```python
from build123d import *

# Parameters (mm, degrees)
F0_R     = 100.5
F1_DEPTH = 107.5
F2_R     = 82
F3_DEPTH = 40
F5_DEPTH = 42.6


with BuildPart() as f1:
    # F0 (on Top) → F1 (new body)
    with BuildSketch(Plane.XY):
        Circle(F0_R)
    extrude(amount=F1_DEPTH)

    # F2 (on face) → F3 (join)
    with BuildSketch(Plane.XY.offset(107.5)):
        Circle(F2_R)
    extrude(amount=F3_DEPTH)

    # F4 (on face) → F5 (join)
    with BuildSketch(Plane(origin=(0, 0, 0), x_dir=(1, 0, 0), z_dir=(0, 0, -1))):
        with BuildLine():
            ThreePointArc((-2.4, 10.847677), (-6.955864, -8.663028), (11.11, 0))
            ThreePointArc((11.11, 0), (8.663028, 6.955864), (2.4, 10.847677))
            Line((2.4, 10.847677), (2.4, 8.46))
            Line((2.4, 8.46), (0, 8.46))
            Line((0, 8.46), (-2.4, 8.46))
            Line((-2.4, 8.46), (-2.4, 10.847677))
        make_face()
        with BuildLine():
            ThreePointArc((5.555, 0), (-3.927978, -3.927978), (0, 5.555))
            ThreePointArc((0, 5.555), (3.927978, 3.927978), (5.555, 0))
        make_face(mode=Mode.SUBTRACT)
    extrude(amount=F5_DEPTH)


solid = f1.part
```
Here's how the part is built. I have some questions about the finished solid (model axes, mm). A direction names the side the tool comes from. Coordinates: 2 decimals unless noted, no trailing zeros. Order: outer loops, then holes, each group sorted by start corner. A loop starts at its lowest first (then second) coordinate and runs counter-clockwise, first axis right, second up.
1) Which directions (+Z, -Z, +X, -X, +Y, -Y) give clear straight access to the entire face, cutting with the end or side of a thin tool? Please do faces 1 (the face through (0, 0, 0)), 2 (the face through (-3, -5, -42.6)), 3 (the face through (-82.4, 0.5, 107.5)).
2) Will these pins go through, and if not, where does the flat tip stop? pin 1 (2 mm diameter, centred on x = -58, z = 60.5, fed in from -Y); pin 2 (5.5 mm diameter, centred on x = 0.5, z = -19, fed in from -Y); pin 3 (4 mm diameter, centred on x = -2, y = 77, fed in from -Z).
3) Imagine slicing it at C-C on z = 26.5. List the corners of the cut face in (x, y) for me, and give its area (3 significant figures).
4) I need wall thicknesses on line 1 (Z direction, x = -34, y = 61); line 2 (Z direction, x = 57, y = 70); line 3 (X direction, y = 70, z = 110). Which ranges of each line are inside material? Lowest first, please.
5) Imagine slicing it at A-A on x = -50. List the corners of the cut face in (y, z) for me.
6) Imagine slicing it at B-B on y = -42. List the corners of the cut face in (x, z) for me.
Response values:
1. face 1: -Z
1. face 2: -Z, +X, -X, +Y, -Y
1. face 3: +Z
2. pin 1: stops at y = -82.77
2. pin 2: stops at y = -10.85
2. pin 3: stops at z = 0
3. outline: circle Ø201 at (0, 0)
3. area: 31,700 mm2
4. line 1: z = 0 to 147.5
4. line 2: z = 0 to 107.5
4. line 3: x = -42.71 to 42.71
5. outline: (-87.18, 0) - (87.18, 0) - (87.18, 107.5) - (64.99, 107.5) - (64.99, 147.5) - (-64.99, 147.5) - (-64.99, 107.5) - (-87.18, 107.5) - close
6. outline: (-91.3, 0) - (91.3, 0) - (91.3, 107.5) - (70.43, 107.5) - (70.43, 147.5) - (-70.43, 147.5) - (-70.43, 107.5) - (-91.3, 107.5) - close
